Drawing for the job (mm, zero at the part's lowest x, y, z). A direction names the side the tool comes from. Give positions to 0.01 mm unless a question says otherwise; leave off trailing zeros. Order: outer loops, then holes, each group sorted by start corner. A loop starts at its lowest first (then second) coordinate and runs counter-clockwise, first axis right, second up. Notation, with made-up numbers: (88, 87.5) -> (95, 87.5) arc R19 ccw to (95, 110.5) -> close; hole circle Ø6 at (49, 6.5). An arc over 180 degrees is marked (long way). Use a Markdown table: item, result. Add a question column.
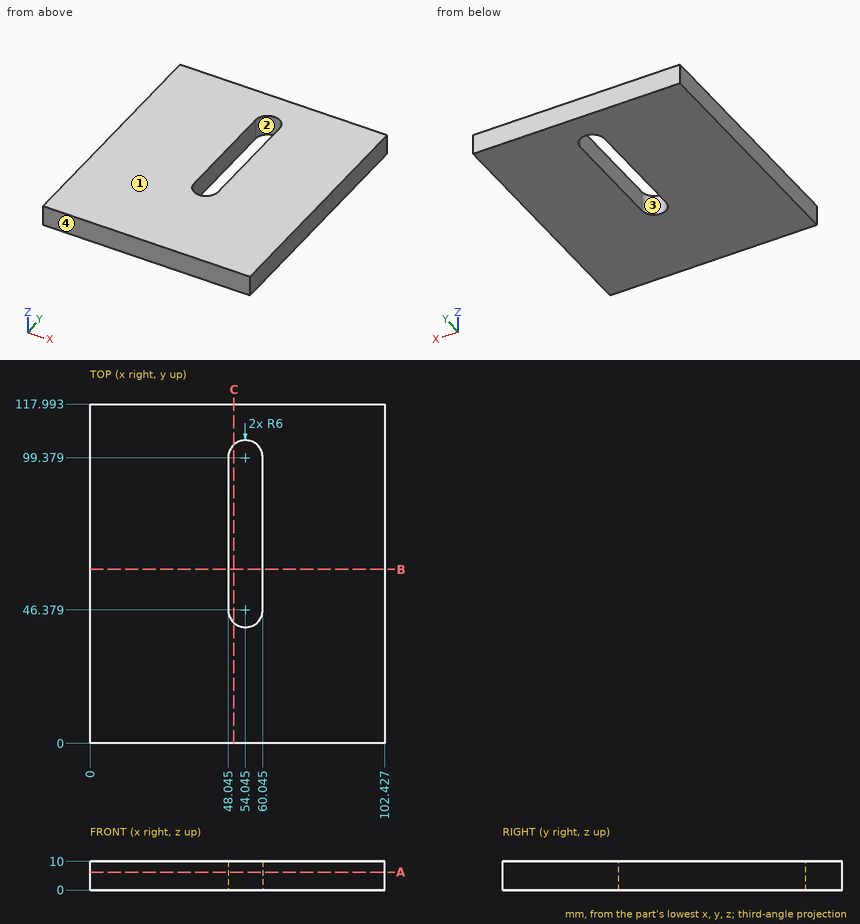
(1) Band-saw the part on A-A on z = 6.25. Give the cut face in (x, y) (1 decimal), plus the area to 3 significant figures.
(2) Mould opens along X. For the marked faces 3 and 4 say: released by +X, released by -X, zero draft, split by the parting line, or undercut.
(3) Band-saw the part on B-B on y = 60.5. Give the cut face in (x, z) (1 decimal), plus the area to 3 significant figures.
(4) Band-saw the part on C-C on x = 50. Give the cut face in (y, z).
(5) Tool access for the marked faces 1 and 2: list every direction of +Z, -Z, +X, -X, +Y, -Y with a clear straight run to the whole face (end or side of a thin tool).
(6) Wall check: probe 1 along X at (y, z) = (95.5, 1.5) (1 decimal); probe 2 along Y at (x, z) = (57.5, 8) (1 decimal); probe 3 along Y at (x, z) = (53.5, 3.25). Give the ranges that are in metal, low to high.
Response:
| question | item | result |
|---|---|---|
| 1 | outline | (0, 0) -> (102.4, 0) -> (102.4, 118) -> (0, 118) -> close; hole (48, 46.4) arc R6 ccw to (60, 46.4) -> (60, 99.4) arc R6 ccw to (48, 99.4) -> close |
| 1 | area | 11,300 mm² |
| 2 | face 3 | undercut |
| 2 | face 4 | zero draft |
| 3 | outline | (0, 0) -> (48, 0) -> (48, 10) -> (0, 10) -> close; (60, 0) -> (102.4, 0) -> (102.4, 10) -> (60, 10) -> close |
| 3 | area | 904 mm² |
| 4 | outline | (0, 0) -> (41.95, 0) -> (41.95, 10) -> (0, 10) -> close; (103.81, 0) -> (117.99, 0) -> (117.99, 10) -> (103.81, 10) -> close |
| 5 | face 1 | +Z, +X, -X, +Y, -Y |
| 5 | face 2 | +Z, -Z |
| 6 | probe 1 | x = 0 to 48, 60 to 102.4 |
| 6 | probe 2 | y = 0 to 41.5, 104.3 to 118 |
| 6 | probe 3 | y = 0 to 40.4, 105.35 to 117.99 |
